from build123d import *

# Parameters (mm, degrees)
EXTRUDE_1_DEPTH        = 1.5
SKETCH_3_R             = 1.1
CUT_EXTRUDE_1_DEPTH    = 5
EXTRUDE_2_DEPTH        = 6.9
SWEEP_1_PROFILE_R      = 1.6
CUT_EXTRUDE_START      = -7.8
CUT_EXTRUDE_5_DEPTH    = 7.8
EXTRUDE_START          = -0.8
SKETCH_81_W            = 5
SKETCH_81_H            = 5
SKETCH_81_R            = 1.1
EXTRUDE_8_DEPTH        = 1.9
FILLET_1_R             = 2
FILLET_1_OF_MIRROR_1_R = 2
SKETCH_83_W            = 6.9
SKETCH_83_H            = 14.5
EXTRUDE_10_DEPTH       = 1


with BuildPart() as part:
    # 草图2 → 凸台-拉伸1 (new body)
    with BuildSketch(Plane(origin=(0, 0, 0), x_dir=(1, 0, 0), z_dir=(0, 1, 0))):
        with BuildLine():
            Line((-4.95, 3.45), (7.45, 3.45))
            Line((7.45, 3.45), (7.45, -3.45))
            Line((7.45, -3.45), (-4.95, -3.45))
            ThreePointArc((-4.95, -3.45), (-6.717766953, -2.717766953), (-7.45, -0.95))
            Line((-7.45, -0.95), (-7.45, 0.95))
            ThreePointArc((-7.45, 0.95), (-6.717766953, 2.717766953), (-4.95, 3.45))
        make_face()
    extrude(amount=EXTRUDE_1_DEPTH)

    # 草图3 → 切除-拉伸1 (cut)
    with BuildSketch(Plane(origin=(0, 1.5, 0), x_dir=(1, 0, 0), z_dir=(0, 1, 0))):
        with Locations(Location((-4.95, 0, 0), (0, 0, 270))):
            Circle(SKETCH_3_R)
    extrude(amount=-CUT_EXTRUDE_1_DEPTH, mode=Mode.SUBTRACT)

    # 草图5 → 凸台-拉伸2 (add)
    with BuildSketch(Plane(origin=(0, 0, -3.45), x_dir=(-1, 0, 0), z_dir=(0, 0, -1))):
        Polygon((2.45, 1.5), (2.45, 14.5), (-7.45, 20.686206584), (-7.45, 1.5), align=None)
    extrude(amount=-EXTRUDE_2_DEPTH)

    # 切除-扫描1: sweep along a path in 草图7
    with BuildLine(Plane.XY) as sweep_1_path:
        Line((-6.203786906, 5.079303189), (11.626887116, 16.221144909))
    # 切除-扫描1 profile (on start of the path) → 切除-扫描1 (sweep, cut)
    with BuildSketch(Plane(origin=(-6.203786906, 5.079303189, 0), x_dir=(-0.529919264233206, 0.8480480961564254, 0), z_dir=(0.8480480961564254, 0.529919264233206, 0))):
        Circle(SWEEP_1_PROFILE_R)
    sweep(path=sweep_1_path.line, mode=Mode.SUBTRACT)

    # 草图80 → 切除-拉伸5 (cut)
    with BuildSketch(Plane(origin=(0, 1.5, 0), x_dir=(1, 0, 0), z_dir=(0, 1, 0)).offset(CUT_EXTRUDE_START)):
        with BuildLine():
            Line((-4.95, -3.45), (-2.45, -3.45))
            Line((-2.45, -3.45), (-2.45, 3.45))
            Line((-2.45, 3.45), (-4.95, 3.45))
            ThreePointArc((-4.95, 3.45), (-6.717766953, 2.717766953), (-7.45, 0.95))
            Line((-7.45, 0.95), (-7.45, -0.95))
            ThreePointArc((-7.45, -0.95), (-6.717766953, -2.717766953), (-4.95, -3.45))
        make_face()
    extrude(amount=CUT_EXTRUDE_5_DEPTH, mode=Mode.SUBTRACT)

    # 草图81 → 凸台-拉伸8 (add)
    with BuildSketch(Plane.XZ.offset(EXTRUDE_START)):
        with Locations((2.5, 5.95)):
            Rectangle(SKETCH_81_W, SKETCH_81_H)
        with Locations(Location((2.5, 5.95, 0), (0, 0, 270))):
            Circle(SKETCH_81_R, mode=Mode.SUBTRACT)
    extrude_8 = extrude(amount=-EXTRUDE_8_DEPTH)

    # 圆角1
    fillet_1_edges = [part.edges().sort_by_distance(p)[0] for p in [
        (5, 1.75, 8.45),
        (0, 1.75, 8.45),
    ]]
    fillet(fillet_1_edges, radius=FILLET_1_R)

    # 镜向1: 凸台-拉伸8 across plane
    add(extrude_8.mirror(Plane.XY))

    # 圆角1 of 镜向1
    fillet_1_of_mirror_1_edges = [part.edges().sort_by_distance(p)[0] for p in [
        (5, 1.75, -8.45),
        (0, 1.75, -8.45),
    ]]
    fillet(fillet_1_of_mirror_1_edges, radius=FILLET_1_OF_MIRROR_1_R)

    # 草图83 → 凸台-拉伸10 (add)
    with BuildSketch(Plane.ZY.offset(2.45)):
        with Locations((0, 7.25)):
            Rectangle(SKETCH_83_W, SKETCH_83_H)
    extrude(amount=-EXTRUDE_10_DEPTH)


solid = part.part
Here's how the part is built. I have some questions about the finished solid (model axes, mm). A direction names the side the tool comes from. Round coordinates to 2 decimals unless told otherwise and drop trailing zeros. Order: outer loops, then holes, each group sorted by start corner. A loop starts at its lowest first (then second) coordinate and runs counter-clockwise, first axis right, second up. Notation, with made-up numbers: (-3, 57.25) -> (2, 57.25) arc R34 cw to (2, 93.25) -> close; hole circle Ø6 at (-7, 40.5). An arc over 180 degrees is marked (long way). Return JSON: item names as keys, results as strings.
Q1. For pin 1 Ø1.5 at (y, z) = (2, -4.5) entering from +X; pin 2 Ø2.5 at (x, z) = (2.5, 5.5) entering from -Y; pin 3 Ø3 at (x, y) = (3.5, 15.5) entering from -Z; pin 4 Ø1.8 at (x, z) = (2.5, -5.95) entering from +Y, each with a flat end and sliding along its axis, tell me the tip position at first contact or that it passes through.
Filled sheet:
{"pin 1": "stops at x = 5", "pin 2": "stops at y = 0.8", "pin 3": "stops at z = -3.45", "pin 4": "passes through"}
Q2. If we section it at C-C on x = 1.75: Give the number of separate pieces and of enclosed holes in the cut face, plus the area to 4 significant figures.
Filled sheet:
{"separate pieces": "3", "enclosed holes": "1", "area": "121.5 mm^2"}
Q3. If we mould it in two halves opening along X, with no side actions, what happens to faces 1 (the flat face through (3, 0, 0)), 2 (the flat face through (5, 2, 5)), 3 (the flat face through (0, 2, -5)), 4 (the cylindrical face through (2.55, 1.74, -7.05))? For each: released by +X, released by -X, zero draft, split by the parting line, or undercut.
Filled sheet:
{"face 1": "zero draft", "face 2": "released by +X", "face 3": "released by -X", "face 4": "undercut"}
Q4. If we section it at B-B on y = 5: List the corners of the cut face in (x, z) for me, plus the area to 3 significant figures.
Filled sheet:
{"outline": "(-2.45, -3.45) -> (7.45, -3.45) -> (7.45, 3.45) -> (-2.45, 3.45) -> close", "area": "68.3 mm^2"}
Q5. Which directions (+Z, -Z, +X, -X, +Y, -Y) give clear straight access to the entire face, cutting with the end or side of a thin tool? Please do faces 5 (the flat face through (5, 2, -5)), 6 (the flat face through (1, 2.7, -6)), 7 (the flat face through (1, 0.8, 6)), 8 (the flat face through (1, 2.7, 6)).
Filled sheet:
{"face 5": "-Z, +X, +Y, -Y", "face 6": "-Z, +X, -X, +Y", "face 7": "+Z, +X, -X, -Y", "face 8": "+Z, +X, -X, +Y"}
Q6. If we section it at A-A on z = 5.95: List the corners of the cut face in (x, y) for me, plus the area to 3 significant figures.
Filled sheet:
{"outline": "(0, 0.8) -> (1.4, 0.8) -> (1.4, 2.7) -> (0, 2.7) -> close; (3.6, 0.8) -> (5, 0.8) -> (5, 2.7) -> (3.6, 2.7) -> close", "area": "5.32 mm^2"}
Q7. I need wall thicknesses on line 1 along X through (y, z) = (2.2, 5.95); line 2 along Z through (x, y) = (0.5, 12.5); line 3 along Y through (x, z) = (2.75, -1). Which ranges of each line are inside material? Lowest first, please. Write a range as from..to.
Filled sheet:
{"line 1": "x = 0..1.4, 3.6..5", "line 2": "z = -3.45..3.45", "line 3": "y = 0..9.2, 12.15..17.75"}
